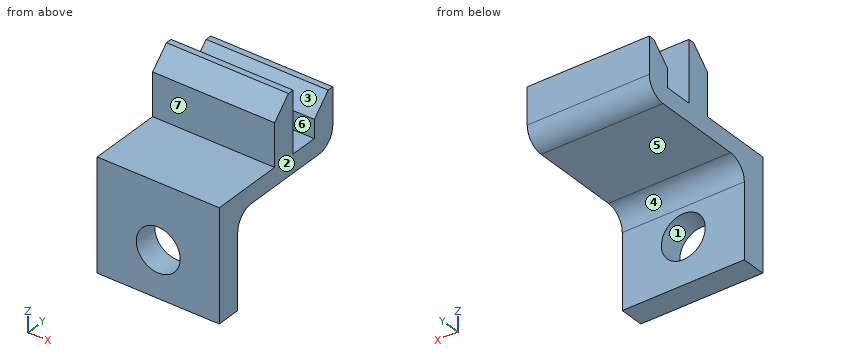
from build123d import *

# Parameters (mm, degrees)
BOSS_EXTRUDE1_DEPTH     = 5
SKETCH2_R               = 1.8
CUT_EXTRUDE1_DEPTH      = 8.15
CUT_EXTRUDE1_DEPTH_BACK = 6.15
CHAMFER2_SIZE           = 1.5
FILLET1_R               = 1.5


with BuildPart() as part:
    # Sketch1 → Boss-Extrude1 (new body, symmetric)
    with BuildSketch(Plane(origin=(0, 0, 0), x_dir=(0, 0, -1), z_dir=(1, 0, 0))):
        Polygon((-8.3, 5.15), (-3.8, 5.15), (-3.8, -5.15), (3.8, -5.15), (3.8, -7.15), (-5.3, -7.15), (-5.3, -1.15), (-10.3, -1.15), (-10.3, 0.85), (-5.3, 0.85), (-5.3, 3.15), (-8.3, 3.15), align=None)
    extrude(amount=BOSS_EXTRUDE1_DEPTH, both=True)

    # Sketch2 → Cut-Extrude1 (cut, two sides)
    with BuildSketch(Plane(origin=(0, 0, 5.3), x_dir=(1, 0, 0), z_dir=(0, -1, 0))) as cut_extrude1_sk:
        with Locations((0, -5.3)):
            Circle(SKETCH2_R)
    extrude(amount=CUT_EXTRUDE1_DEPTH, mode=Mode.SUBTRACT)
    extrude(cut_extrude1_sk.sketch, amount=-CUT_EXTRUDE1_DEPTH_BACK, mode=Mode.SUBTRACT)

    # Chamfer2
    chamfer2_edges = [part.edges().sort_by_distance(p)[0] for p in [
        (0, -1.15, 10.3),
        (0, 3.15, 8.3),
    ]]
    chamfer(chamfer2_edges, length=CHAMFER2_SIZE)

    # Fillet1
    fillet1_edges = [part.edges().sort_by_distance(p)[0] for p in [
        (0, 5.15, 3.8),
        (0, -5.15, 3.8),
    ]]
    fillet(fillet1_edges, radius=FILLET1_R)


solid = part.part
Geometry: final body of the model. Coordinates: model frame, mm. Face numbers are marked on the shaded views. A direction names the side the tool comes from. Give positions to 0.01 mm unless a question says otherwise; leave off trailing zeros. Order: outer loops, then holes, each group sorted by start corner. A loop starts at its lowest first (then second) coordinate and runs counter-clockwise, first axis right, second up. Notation, with made-up numbers: (-13.5, 41) -> (8.5, 41) arc R7 ccw to (8.5, 54) -> close; hole circle Ø11 at (17.5, 17). An arc over 180 degrees is marked (long way). Put each result on its own line as item: value.
Q1. Section C-C, the plane x = 3.5. Return loops of the section in (y, z).
Here are the results:
outline: (-7.15, -3.8) -> (-5.15, -3.8) -> (-5.15, 2.3) arc R1.5 cw to (-3.65, 3.8) -> (3.65, 3.8) arc R1.5 ccw to (5.15, 5.3) -> (5.15, 8.3) -> (4.65, 8.3) -> (3.15, 6.8) -> (3.15, 5.3) -> (0.85, 5.3) -> (0.85, 10.3) -> (0.35, 10.3) -> (-1.15, 8.8) -> (-1.15, 5.3) -> (-7.15, 5.3) -> close
Q2. Reachability of the marked faces 5, 6 and 7 from +Z, -Z, +X, -X, +Y, -Y: full face, straight path, thin tool, end or side. Return the list, or none.
Here are the results:
face 5: -Z, +X, -X, +Y
face 6: +Z, +X, -X
face 7: +Z, +X, -X, -Y
Q3. Material intervals for L1, parallel to X at y = -5.75, z = 0; L2, parallel to Z at x = 0, y = -6.2; L3, parallel to Y at x = 1.5, z = 6.75, sorted ascending.
Here are the results:
L1: x = -5 to -1.8, 1.8 to 5
L2: z = -3.8 to -1.8, 1.8 to 5.3
L3: y = -1.15 to 0.85, 3.15 to 5.15
Q4. Section A-A, the plane x = 0. Return loops of the section in (y, z), then the cut area to 3 significant figures.
Here are the results:
outline: (-7.15, -3.8) -> (-5.15, -3.8) -> (-5.15, -1.8) -> (-7.15, -1.8) -> close; (-7.15, 1.8) -> (-5.15, 1.8) -> (-5.15, 2.3) arc R1.5 cw to (-3.65, 3.8) -> (3.65, 3.8) arc R1.5 ccw to (5.15, 5.3) -> (5.15, 8.3) -> (4.65, 8.3) -> (3.15, 6.8) -> (3.15, 5.3) -> (0.85, 5.3) -> (0.85, 10.3) -> (0.35, 10.3) -> (-1.15, 8.8) -> (-1.15, 5.3) -> (-7.15, 5.3) -> close
area: 40.2 mm^2
Q5. Section D-D, the plane y = -2.25. Return loops of the section in (x, z).
Here are the results:
outline: (-5, 3.8) -> (5, 3.8) -> (5, 5.3) -> (-5, 5.3) -> close
Q6. Draft query along Z for the marked faces 1, 2, 3 and 4. Return one class per face: released by +Z, released by -Z, zero draft, split by the parting line, or undercut.
Here are the results:
face 1: undercut
face 2: zero draft
face 3: released by +Z
face 4: released by -Z
Q7. Pin query (flat end, axial travel): pin 1 (3 mm diameter, centred on x = 0.5, z = -0.5, fed in from +Y); pin 2 (4 mm diameter, centred on x = -0.5, y = -3, fed in from +Z); pin 3 (4 mm diameter, centred on x = -0.5, y = 3, fed in from +Z); pin 4 (6 mm diameter, centred on x = 2, y = -2.5, fed in from -Z). Return the tip coordinate at first contact, or that it passes through.
Here are the results:
pin 1: stops at y = -5.15
pin 2: stops at z = 8.95
pin 3: stops at z = 8.3
pin 4: stops at z = -3.8
Q8. Section B-B, the plane z = 0. Return loops of the section in (x, y).
Here are the results:
outline: (-5, -7.15) -> (-1.8, -7.15) -> (-1.8, -5.15) -> (-5, -5.15) -> close; (1.8, -7.15) -> (5, -7.15) -> (5, -5.15) -> (1.8, -5.15) -> close
